The model under review builds one solid part; all positions refer to its coordinate system, in mm. Face numbers are marked on the shaded views. A direction names the side the tool comes from. Round coordinates to 2 decimals unless told otherwise and drop trailing zeros. Loops run counter-clockwise (first coordinate to the right, second up) from the corner with the lowest first, then second, coordinate; pieces in that order, holes last. Notation, with made-up numbers: M 8,35.25 L 12,35.25 A23 cw 12,60.25 Z; hole C -33,-15.75 d3. An arc over 180 degrees is marked long. Return JSON: item names as keys, results as strings. Group by question number.
Q1. To check wall thickness, follow line 1 along X through (y, z) = (19.5, -2.5); line 2 along Y through (x, z) = (-127.75, 3.25); line 3 along X through (y, z) = (22, 5). State the ranges of each line that lie inside material, in increasing order.
Q2. Draft analysis for pull direction X (two halves, no side actions). For the marked faces 1, 2, 3 and 4, state which applies: pulls with the +X half, pulls with the -X half, needs draft (parallel to the pull), parting line crosses it, or undercut.
Q3. Consider section A-A (z = 5.25). Count the separate pieces of the cut face and the enclosed holes in it, and give its area (3 significant figures).
Q4. Consider section D-D (x = -113.5). State the section outline as (y, z) points.
Q5. Consider section B-B (x = -128). State the section outline as (y, z) points, and give its area (3 significant figures).
Q6. Consider section C-C (y = 35.5). State the section outline as (x, z) points, and give its area (3 significant figures).
Q7. For the marked faces 5, 6 and 7, list the 3-axis set-ups (+Z, -Z, +X, -X, +Y, -Y) from which the entire face can be reached by the end or side of a thin tool; tool diameter is ignored.
Q8. Clearance check with flat-ended pins moving along their axes: pin 1 Ø8 at (x, z) = (-119.23, 5) entering from -Y; pin 2 Ø1.1 at (y, z) = (42.5, 5.5) entering from -X; pin 3 Ø9.5 at (y, z) = (33, -3.5) entering from +X; pin 4 Ø4 at (x, y) = (-131.23, 17.7) entering from -Z. State where each tip first meets the part, or that it passes through.
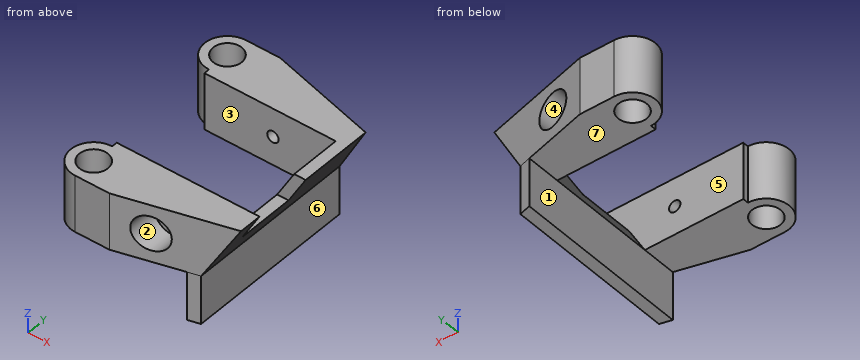
from build123d import *

# Parameters (mm, degrees)
CROQUIS1_R              = 2.5
SALIENTE_EXTRUIR1_DEPTH = 10
CROQUIS2_R              = 1
CORTAR_EXTRUIR1_DEPTH   = 4
SALIENTE_EXTRUIR2_DEPTH = 13.5
CROQUIS4_R              = 3
CORTAR_EXTRUIR2_DEPTH   = 1
SALIENTE_EXTRUIR3_START = 5
CROQUIS6_R              = 3
SALIENTE_EXTRUIR3_DEPTH = 5
CORTAR_EXTRUIR3_DEPTH   = 10
SALIENTE_EXTRUIR4_DEPTH = 8.5
CROQUIS5_W              = 2
CROQUIS5_H              = 10
CORTAR_EXTRUIR4_DEPTH   = 6


with BuildPart() as part:
    # Croquis1 → Saliente-Extruir1 (new body)
    with BuildSketch(Plane.XY):
        with BuildLine():
            Line((-106.231635218, 22.700651543), (-131.231635218, 22.700651543))
            Line((-131.231635218, 22.700651543), (-131.231635218, 21.700651543))
            ThreePointArc((-131.231635218, 21.700651543), (-135.231635218, 17.700651543), (-131.231635218, 13.700651543))
            Line((-131.231635218, 13.700651543), (-125.231635218, 13.700651543))
            Line((-125.231635218, 13.700651543), (-125.231635218, 18.700651543))
            Line((-125.231635218, 18.700651543), (-106.231635218, 18.700651543))
            Line((-106.231635218, 18.700651543), (-106.231635218, 22.700651543))
        make_face()
        with Locations((-131.231635218, 17.700651543)):
            Circle(CROQUIS1_R, mode=Mode.SUBTRACT)
    extrude(amount=SALIENTE_EXTRUIR1_DEPTH)

    # Croquis2 → Cortar-Extruir1 (cut)
    with BuildSketch(Plane.XZ.offset(-18.700651543)):
        with Locations(Location((-119.231635218, 5, 0), (0, 0, 270))):
            Circle(CROQUIS2_R)
        Polygon((-106.231635218, 0), (-106.231635218, 10), (-112.00513791, 0), align=None)
    extrude(amount=-CORTAR_EXTRUIR1_DEPTH, mode=Mode.SUBTRACT)

    # Croquis3 → Saliente-Extruir2 (add)
    with BuildSketch(Plane.XZ.offset(-18.700651543)):
        Polygon((-106.231635218, 10), (-108.231635218, 10), (-114.00513791, 0), (-112.00513791, 0), align=None)
    extrude(amount=-SALIENTE_EXTRUIR2_DEPTH)

    # Croquis4 → Cortar-Extruir2 (cut)
    with BuildSketch(Plane.XZ.offset(-18.700651543)):
        with Locations(Location((-119.231635218, 5, 0), (0, 0, 270))):
            Circle(CROQUIS4_R)
    extrude(amount=-CORTAR_EXTRUIR2_DEPTH, mode=Mode.SUBTRACT)

    # Croquis6 → Saliente-Extruir3 (add)
    with BuildSketch(Plane.XZ.offset(-18.700651543).offset(SALIENTE_EXTRUIR3_START)):
        Polygon((-106.231635218, 10), (-125.231635218, 10), (-125.231635218, 0), (-112.00513791, 0), align=None)
        with Locations(Location((-119.231635218, 5, 0), (0, 0, 270))):
            Circle(CROQUIS6_R, mode=Mode.SUBTRACT)
    extrude(amount=-SALIENTE_EXTRUIR3_DEPTH)

    # Croquis7 → Cortar-Extruir3 (cut)
    with BuildSketch(Plane.XY.offset(10)):
        Polygon((-106.231635218, 18.700651543), (-106.231635218, 13.700651543), (-125.231635218, 13.700651543), align=None)
    extrude(amount=-CORTAR_EXTRUIR3_DEPTH, mode=Mode.SUBTRACT)

    # Croquis8 → Saliente-Extruir4 (add)
    with BuildSketch(Plane(origin=(0, 0, 0), x_dir=(-1, 0, 0), z_dir=(0, 0, -1))):
        Polygon((112.00513791, 17.181308729), (112.00513791, 32.200651543), (114.00513791, 32.200651543), (114.00513791, 16.65499294), align=None)
    extrude(amount=SALIENTE_EXTRUIR4_DEPTH)

    # Simetría1: part across plane


with BuildPart() as part_1:
    add(part.part)
    add(part.part.mirror(Plane(origin=(0, 32.200651543, 0), x_dir=(0, 0, 1), z_dir=(0, -1, 0))))

    # Croquis5 → Cortar-Extruir4 (cut, along a direction that is not the sketch's normal)
    with BuildSketch(Plane.XY.offset(10)):
        with Locations((-107.231635218, 27.700651543)):
            Rectangle(CROQUIS5_W, CROQUIS5_H)
    extrude(amount=-CORTAR_EXTRUIR4_DEPTH, dir=(0.49999999999999506, 0, 0.8660254037844416), mode=Mode.SUBTRACT)


solid = part_1.part
Values:
{
 "1": {"line 1": "x = -114.01 to -112.01", "line 2": "y = 13.7 to 22.7, 41.7 to 50.7", "line 3": "x = -131.23 to -120.23, -118.23 to -109.12"},
 "2": {"face 1": "pulls with the -X half", "face 2": "undercut", "face 3": "needs draft", "face 4": "undercut"},
 "3": {"separate pieces": "4", "enclosed holes": "2", "area": "296 mm2"},
 "4": {"outline": "M 16.79,-8.5 L 47.61,-8.5 L 47.61,10 L 41.7,10 L 41.7,0.87 L 22.7,0.87 L 22.7,10 L 16.79,10 Z"},
 "5": {"outline": "M 13.7,0 L 22.7,0 L 22.7,10 L 13.7,10 Z; M 41.7,0 L 50.7,0 L 50.7,10 L 41.7,10 Z", "area": "180 mm2"},
 "6": {"outline": "M -114.01,-8.5 L -112.01,-8.5 L -112.01,0 L -106.23,10 L -108.23,10 L -114.01,0 Z", "area": "37.0 mm2"},
 "7": {"face 5": "+Z, -X", "face 6": "-Z, +X, +Y, -Y", "face 7": "-Z, -X, +Y, -Y"},
 "8": {"pin 1": "stops at y = 14.23", "pin 2": "stops at x = -132.87", "pin 3": "stops at x = -111.28", "pin 4": "passes through"}
}
